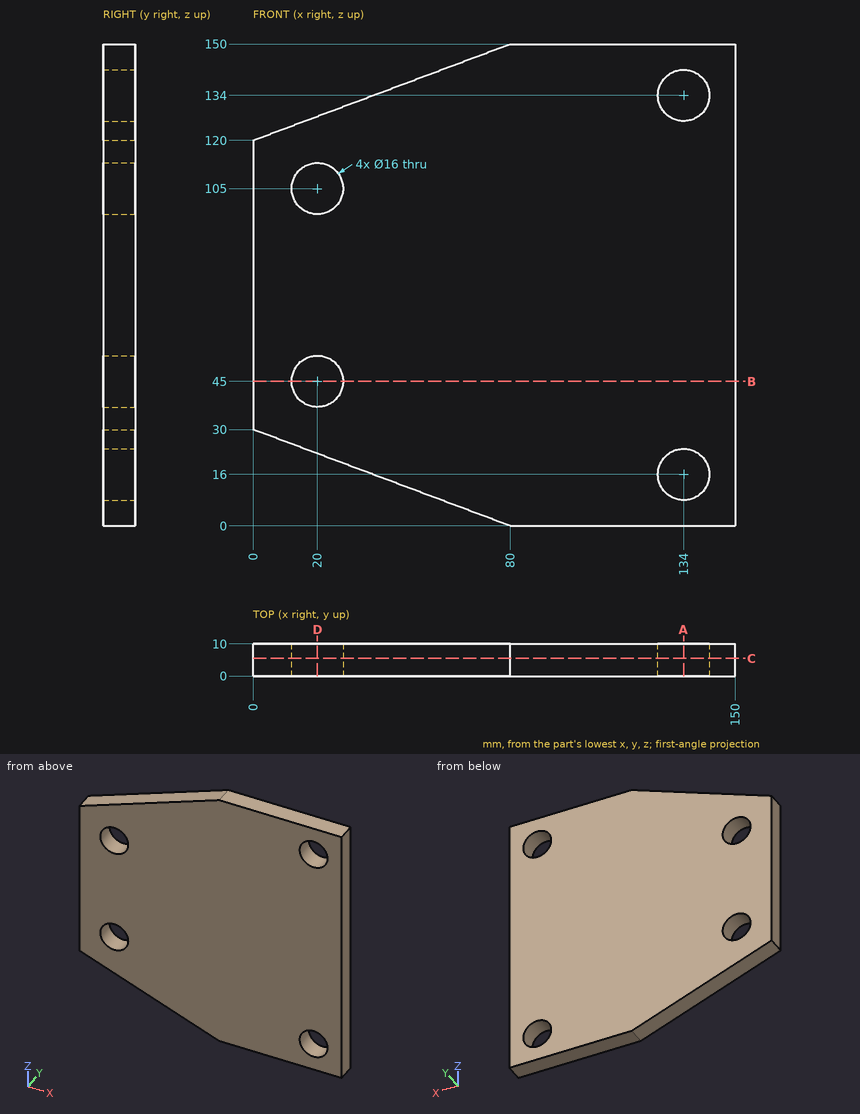
Design review of the part shown in the three views and the two pictorial views. Dimensions are in mm from the part's minimum x, y and z. Give positions to 0.01 mm unless a question says otherwise; leave off trailing zeros. Write each loop counter-clockwise with the first axis right and the second up, starting at its lowest first coordinate (ties: lowest second). Pieces come first, ordered by that corner, then holes. Notation, with made-up numbers: (66, 52) -> (93, 52) arc R21 ccw to (93, 90) -> close; hole circle Ø9 at (-14.75, -23.75). An arc over 180 degrees is marked (long way). Answer in a Markdown table with one row per item.
1) Add section B-B on z = 45. State the section outline as (x, y) points.
Worked answers:
| item | result |
|---|---|
| outline | (0, 0) -> (12, 0) -> (12, 10) -> (0, 10) -> close; (28, 0) -> (150, 0) -> (150, 10) -> (28, 10) -> close |
2) Add section C-C on y = 5.5. State the section outline as (x, z) points.
Worked answers:
| item | result |
|---|---|
| outline | (0, 30) -> (80, 0) -> (150, 0) -> (150, 150) -> (80, 150) -> (0, 120) -> close; hole circle Ø16 at (20, 45); hole circle Ø16 at (20, 105); hole circle Ø16 at (134, 16); hole circle Ø16 at (134, 134) |
3) Add section D-D on x = 20. State the section outline as (y, z) points.
Worked answers:
| item | result |
|---|---|
| outline | (0, 22.5) -> (10, 22.5) -> (10, 37) -> (0, 37) -> close; (0, 53) -> (10, 53) -> (10, 97) -> (0, 97) -> close; (0, 113) -> (10, 113) -> (10, 127.5) -> (0, 127.5) -> close |
4) For L1, parallel to Z at x = 134, y = 5.5; L2, parallel to Z at x = 20, y = 6.5; L3, parallel to X at y = 2.75, z = 45, list the stretches that pass through material, from the lowest coordinate up. Write a range as [from, to].
Worked answers:
| item | result |
|---|---|
| L1 | [0, 8], [24, 126], [142, 150] |
| L2 | [22.5, 37], [53, 97], [113, 127.5] |
| L3 | [0, 12], [28, 150] |
5) Clearance check with flat-ended pins moving along their axes: P1, Ø3, axis at x = 25.5, y = 5.5, coming from the +Z side (3 decimals); P2, Ø1, axis at x = 18, y = 8, coming from the +Z side. State where each tip first meets the part, or that it passes through.
Worked answers:
| item | result |
|---|---|
| P1 | z = 130.125 |
| P2 | z = 126.94 |
6) Add section A-A on x = 134. State the section outline as (y, z) points.
Worked answers:
| item | result |
|---|---|
| outline | (0, 0) -> (10, 0) -> (10, 8) -> (0, 8) -> close; (0, 24) -> (10, 24) -> (10, 126) -> (0, 126) -> close; (0, 142) -> (10, 142) -> (10, 150) -> (0, 150) -> close |
